Design review of the part built by this model. Coordinates are the model's own, in mm. A direction names the side the tool comes from. Give positions to 0.01 mm unless a question says otherwise; leave off trailing zeros. Write each loop counter-clockwise with the first axis right and the second up, starting at its lowest first coordinate (ties: lowest second). Pieces come first, ordered by that corner, then holes. Notation, with made-up numbers: (20.25, 75.5) -> (53.25, 75.5) arc R31 cw to (53.25, 100.5) -> close; hole circle Ø4 at (73, -38.75). An arc over 180 degrees is marked (long way). Answer as a JSON object with one key per item and string values.
```python
from build123d import *

# Parameters (mm, degrees)
F0_W     = 176.5
F0_H     = 199.5
F1_DEPTH = 5
F2_W     = 2.5
F2_H     = 83.7
F2_H_2   = 83.8
F3_DEPTH = 25
F4_W     = 15
F4_H     = 21
F5_DEPTH = 2.5
F6_W     = 13.2
F6_H     = 12.4
F7_DEPTH = 2.5
F8_W     = 13.2
F8_H     = 12.4
F8_W_2   = 24
F8_H_2   = 15
F9_DEPTH = 2.5


# Not quite as in the source:
# - a feature names something its author has since deleted; it is built from what else it names


with BuildPart() as f1:
    # F0 (on Top) → F1 (new body)
    with BuildSketch(Plane.XY):
        with Locations((-57.1313334405, 21.2478748113)):
            Rectangle(F0_W, F0_H)
    extrude(amount=F1_DEPTH)

    # F2 (on face) → F3 (join)
    with BuildSketch(Plane.XY.offset(5)):
        Polygon((-141.8813334405, 33.7978748113), (-144.3813334405, 33.7978748113), (-144.3813334405, 31.2978748113), (-113.3813334405, 31.2978748113), (-113.3813334405, 11.2978748113), (-144.3813334405, 11.2978748113), (-144.3813334405, 8.7978748113), (-141.8813334405, 8.7978748113), (-110.8813334405, 8.7978748113), (-110.8813334405, 33.7978748113), align=None)
        with Locations((-143.1313334405, 75.6478748113)):
            Rectangle(F2_W, F2_H)
        Polygon((30.1186665595, 119.9978748113), (-144.3813334405, 119.9978748113), (-144.3813334405, 117.4978748113), (-141.8813334405, 117.4978748113), (27.6186665595, 117.4978748113), (27.6186665595, -75.0021251887), (-141.8813334405, -75.0021251887), (-144.3813334405, -75.0021251887), (-144.3813334405, -77.5021251887), (30.1186665595, -77.5021251887), align=None)
        with Locations((-143.1313334405, -33.1021251887)):
            Rectangle(F2_W, F2_H_2)
    extrude(amount=F3_DEPTH)

    # F4 (on face) → F5 (cut, through all)
    with BuildSketch(Plane(origin=(-113.3813334405, 0, 0), x_dir=(0, -1, 0), z_dir=(-1, 0, 0))):
        with Locations((-21.2978748113, 15.5)):
            Rectangle(F4_W, F4_H)
    extrude(amount=-F5_DEPTH, mode=Mode.SUBTRACT)

    # F6 (on face) → F7 (cut, through all)
    with BuildSketch(Plane(origin=(-144.3813334405, 0, 0), x_dir=(0, -1, 0), z_dir=(-1, 0, 0))):
        with Locations((-72.0978748113, 19.8)):
            Rectangle(F6_W, F6_H)
        with Locations((-42.8978748113, 19.8)):
            Rectangle(F6_W, F6_H)
        with Locations((0.3021251887, 19.8)):
            Rectangle(F6_W, F6_H)
        with Locations((29.5021251887, 19.8)):
            Rectangle(F6_W, F6_H)
    extrude(amount=-F7_DEPTH, mode=Mode.SUBTRACT)

    # F8 (on face) → F9 (cut, through all)
    with BuildSketch(Plane.XZ.offset(77.5021251887)):
        with Locations((-132.7813334405, 19.8)):
            Rectangle(F8_W, F8_H)
        with Locations((-72.3813334405, 18.5)):
            Rectangle(F8_W_2, F8_H_2)
        with Locations((-47.2813334405, 19.8)):
            Rectangle(F8_W, F8_H)
        with Locations((13.1186665595, 18.5)):
            Rectangle(F8_W_2, F8_H_2)
    extrude(amount=-F9_DEPTH, mode=Mode.SUBTRACT)


solid = f1.part
```
(1) We need section B-B, the plane y = 16.5. State the section outline as (x, z) points.
Here are the results:
{"outline": "(-145.38, 0) -> (31.12, 0) -> (31.12, 5) -> (30.12, 5) -> (30.12, 30) -> (27.62, 30) -> (27.62, 5) -> (-145.38, 5) -> close; (-113.38, 26) -> (-110.88, 26) -> (-110.88, 30) -> (-113.38, 30) -> close"}
(2) Clearance check with flat-ended pins moving along their axes: pin 1 (12.5 mm diameter, centred on x = -60, z = 16.5, fed in from -Y); pin 2 (2 mm diameter, centred on y = 77.5, z = 15.5, fed in from +X); pin 3 (4 mm diameter, centred on x = -28, y = 59, fed in from +Z). State where each tip first meets the part, or that it passes through.
Here are the results:
{"pin 1": "stops at y = -77.5", "pin 2": "stops at x = 30.12", "pin 3": "stops at z = 5"}
(3) We need section D-D, the plane x = -4.5. State the section outline as (y, z) points, then the cut area to 3 significant figures.
Here are the results:
{"outline": "(-78.5, 0) -> (121, 0) -> (121, 5) -> (120, 5) -> (120, 30) -> (117.5, 30) -> (117.5, 5) -> (-75, 5) -> (-75, 30) -> (-77.5, 30) -> (-77.5, 5) -> (-78.5, 5) -> close", "area": "1,120 mm²"}
(4) For line 1 along Y through (x, z) = (-115.5, 25.5); line 2 along X through (y, z) = (100.5, 21.25); line 3 along Y through (x, z) = (-129, 16), list the stretches that pass through material, from the lowest coordinate up.
Here are the results:
{"line 1": "y = -77.5 to -75, 8.8 to 11.3, 31.3 to 33.8, 117.5 to 120", "line 2": "x = -144.38 to -141.88, 27.62 to 30.12", "line 3": "y = 8.8 to 11.3, 31.3 to 33.8, 117.5 to 120"}
(5) We need section C-C, the plane y = -49. State the section outline as (x, z) points, then the cut area to 3 significant figures.
Here are the results:
{"outline": "(-145.38, 0) -> (31.12, 0) -> (31.12, 5) -> (30.12, 5) -> (30.12, 30) -> (27.62, 30) -> (27.62, 5) -> (-141.88, 5) -> (-141.88, 30) -> (-144.38, 30) -> (-144.38, 5) -> (-145.38, 5) -> close", "area": "1,010 mm²"}
(6) For faces 1 (the flat face through (-144.381, -32, 12)), 2 (the flat face through (-58, 117.498, 17)), 3 (the flat face through (-58, -77.502, 17)), 4 (the flat face through (-129, 31.298, 17)), list the 3-axis set-ups (+Z, -Z, +X, -X, +Y, -Y) from which the entire face can be reached by the end or side of a thin tool; tool diameter is ignored.
Here are the results:
{"face 1": "+Z, -X, +Y, -Y", "face 2": "+Z", "face 3": "+Z, +X, -X, -Y", "face 4": "+Z, -X"}
(7) We need section A-A, the plane x = -51.5. State the section outline as (y, z) points, then the cut area to 3 significant figures.
Here are the results:
{"outline": "(-78.5, 0) -> (121, 0) -> (121, 5) -> (120, 5) -> (120, 30) -> (117.5, 30) -> (117.5, 5) -> (-75, 5) -> (-75, 13.6) -> (-77.5, 13.6) -> (-77.5, 5) -> (-78.5, 5) -> close; (-77.5, 26) -> (-75, 26) -> (-75, 30) -> (-77.5, 30) -> close", "area": "1,090 mm²"}
(8) The part is to be moulded in two halves that separate along X. For faces 5 (the flat face through (-126, 33.798, 17)), 6 (the flat face through (-144.381, 86, 17)), 7 (the flat face through (30.119, 20, 17)), say which applies: +X half, -X half, draft (parallel to the pull), parting line (faces both ways), or undercut.
Here are the results:
{"face 5": "undercut", "face 6": "-X half", "face 7": "+X half"}
